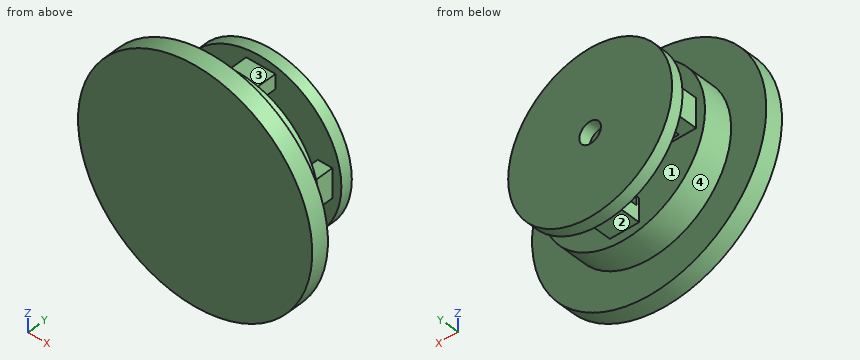
```python
from build123d import *

# Parameters (mm, degrees)
SKETCH_1_R          = 200
EXTRUDE_1_DEPTH     = 30
SKETCH_2_R          = 140
EXTRUDE_2_DEPTH     = 50
SKETCH_4_R          = 1.75
CUT_EXTRUDE_1_DEPTH = 28
SKETCH_7_W          = 25
SKETCH_7_H          = 50
SKETCH_7_W_2        = 50
SKETCH_7_H_2        = 25
EXTRUDE_5_DEPTH     = 43
SKETCH_8_W          = 15
SKETCH_8_H          = 50
SKETCH_8_W_2        = 50
SKETCH_8_H_2        = 15
EXTRUDE_6_DEPTH     = 5
SKETCH_9_R          = 1.75
CUT_EXTRUDE_2_DEPTH = 20
SKETCH_10_R         = 140
EXTRUDE_7_DEPTH     = 20
SKETCH_11_R         = 2.5
CUT_EXTRUDE_3_DEPTH = 20
CUT_EXTRUDE_4_REACH = 318.937
SKETCH_13_R         = 18.5


with BuildPart() as part:
    # 草图1 → 凸台-拉伸1 (new body)
    with BuildSketch(Plane(origin=(0, 0, 0), x_dir=(1, 0, 0), z_dir=(0, 1, 0))):
        with Locations(Location((0, 0, 0), (0, 0, 270))):
            Circle(SKETCH_1_R)
    extrude(amount=EXTRUDE_1_DEPTH)

    # 草图2 → 凸台-拉伸2 (add)
    with BuildSketch(Plane(origin=(0, 30, 0), x_dir=(1, 0, 0), z_dir=(0, 1, 0))):
        with Locations(Location((0, 0, 0), (0, 0, 270))):
            Circle(SKETCH_2_R)
    extrude(amount=EXTRUDE_2_DEPTH)

    # 草图4 → 切除-拉伸1 (cut)
    with BuildSketch(Plane(origin=(0, 80, 0), x_dir=(1, 0, 0), z_dir=(0, 1, 0))):
        with Locations(Location((0, -42.5, 0), (0, 0, 270))):
            Circle(SKETCH_4_R)
        with Locations(Location((-30.0520382, -30.0520382, 0), (0, 0, 270))):
            Circle(SKETCH_4_R)
        with Locations(Location((-42.5, 0, 0), (0, 0, 270))):
            Circle(SKETCH_4_R)
        with Locations(Location((-30.0520382, 30.0520382, 0), (0, 0, 270))):
            Circle(SKETCH_4_R)
        with Locations(Location((0, 42.5, 0), (0, 0, 270))):
            Circle(SKETCH_4_R)
        with Locations(Location((30.0520382, 30.0520382, 0), (0, 0, 270))):
            Circle(SKETCH_4_R)
        with Locations(Location((42.5, 0, 0), (0, 0, 270))):
            Circle(SKETCH_4_R)
        with Locations(Location((30.0520382, -30.0520382, 0), (0, 0, 270))):
            Circle(SKETCH_4_R)
    extrude(amount=-CUT_EXTRUDE_1_DEPTH, mode=Mode.SUBTRACT)

    # 草图7 → 凸台-拉伸5 (add)
    with BuildSketch(Plane(origin=(0, 80, 0), x_dir=(1, 0, 0), z_dir=(0, 1, 0))):
        with Locations((-112.162325809, -2.462481049)):
            Rectangle(SKETCH_7_W, SKETCH_7_H)
        with Locations((2.462481049, -112.162325809)):
            Rectangle(SKETCH_7_W_2, SKETCH_7_H_2)
        with Locations((-2.462481049, 112.162325809)):
            Rectangle(SKETCH_7_W_2, SKETCH_7_H_2)
        with Locations((112.162325809, 2.462481049)):
            Rectangle(SKETCH_7_W, SKETCH_7_H)
    extrude(amount=EXTRUDE_5_DEPTH)

    # 草图8 → 凸台-拉伸6 (add)
    with BuildSketch(Plane(origin=(0, 80, 0), x_dir=(1, 0, 0), z_dir=(0, 1, 0))):
        with Locations((92.162325809, 2.462481049)):
            Rectangle(SKETCH_8_W, SKETCH_8_H)
        with Locations((-2.462481049, 92.162325809)):
            Rectangle(SKETCH_8_W_2, SKETCH_8_H_2)
        with Locations((2.462481049, -92.162325809)):
            Rectangle(SKETCH_8_W_2, SKETCH_8_H_2)
        with Locations((-92.162325809, -2.462481049)):
            Rectangle(SKETCH_8_W, SKETCH_8_H)
    extrude(amount=EXTRUDE_6_DEPTH)

    # 草图9 → 切除-拉伸2 (cut)
    with BuildSketch(Plane(origin=(0, 85, 0), x_dir=(1, 0, 0), z_dir=(0, 1, 0))):
        with Locations(Location((18.656155403, -92.162325809, 0), (0, 0, 270))):
            Circle(SKETCH_9_R)
        with Locations(Location((-11.970984699, -92.162325809, 0), (0, 0, 270))):
            Circle(SKETCH_9_R)
        with Locations(Location((-92.162325809, 11.970984699, 0), (0, 0, 270))):
            Circle(SKETCH_9_R)
        with Locations(Location((-92.162325809, -18.656155403, 0), (0, 0, 270))):
            Circle(SKETCH_9_R)
        with Locations(Location((11.970984699, 92.162325809, 0), (0, 0, 270))):
            Circle(SKETCH_9_R)
        with Locations(Location((-18.656155403, 92.162325809, 0), (0, 0, 270))):
            Circle(SKETCH_9_R)
        with Locations(Location((92.162325809, -11.970984699, 0), (0, 0, 270))):
            Circle(SKETCH_9_R)
        with Locations(Location((92.162325809, 18.656155403, 0), (0, 0, 270))):
            Circle(SKETCH_9_R)
    extrude(amount=-CUT_EXTRUDE_2_DEPTH, mode=Mode.SUBTRACT)

    # 草图10 → 凸台-拉伸7 (add)
    with BuildSketch(Plane(origin=(0, 123, 0), x_dir=(1, 0, 0), z_dir=(0, 1, 0))):
        with Locations(Location((0, 0, 0), (0, 0, 270))):
            Circle(SKETCH_10_R)
    extrude(amount=EXTRUDE_7_DEPTH)

    # 草图11 → 切除-拉伸3 (cut)
    with BuildSketch(Plane(origin=(0, 143, 0), x_dir=(1, 0, 0), z_dir=(0, 1, 0))):
        with Locations(Location((0, 0, 0), (0, 0, 270))):
            Circle(SKETCH_11_R)
    extrude(amount=-CUT_EXTRUDE_3_DEPTH, mode=Mode.SUBTRACT)

    # 草图13 → 切除-拉伸4 (cut, up to next)
    with BuildSketch(Plane(origin=(0, 143, 0), x_dir=(1, 0, 0), z_dir=(0, 1, 0)), mode=Mode.PRIVATE) as cut_extrude_4_sk1:
        with Locations(Location((0, 0, 0), (0, 0, 270))):
            Circle(SKETCH_13_R)
    cut_extrude_4_tool1 = extrude(cut_extrude_4_sk1.sketch, amount=-CUT_EXTRUDE_4_REACH, mode=Mode.PRIVATE) & part.part
    add(cut_extrude_4_tool1.solids().sort_by_distance((0, 143, 0))[0], mode=Mode.SUBTRACT)


solid = part.part
```
Check sheet for the modelled part. Datum: model origin and axes. Units: mm. Face numbers are marked on the shaded views. A direction names the side the tool comes from. Give positions to 0.01 mm unless a question says otherwise; leave off trailing zeros. Loops run counter-clockwise (first coordinate to the right, second up) from the corner with the lowest first, then second, coordinate; pieces in that order, holes last. Notation, with made-up numbers: (18.25, 48.25) - (52.25, 48.25) arc R19 ccw to (52.25, 65.25) - close; hole circle Ø11 at (18, 72.25). An arc over 180 degrees is marked (long way). One line per question, with ' | ' between items. Start each with the question number.
1. Gauge pin test, flat ends, axial feed: pin 1 Ø2.5 at (y, z) = (81.5, 2.5) entering from -X; pin 2 Ø4 at (y, z) = (128.5, 121.5) entering from -X; pin 3 Ø21.5 at (x, y) = (-1, 108.5) entering from +Z. Record the tip position at first contact, or that the pin passes through.
2. Cross-section at A-A, the plane y = 102. Enter the section's corners in (x, z).
3. Cross-section at C-C, the plane x = -54. Enter the section's corners in (y, z).
4. Material ranges on line 1 along Y through (x, z) = (53, -119.5); line 2 along Z through (x, y) = (-23.5, 114.5); line 3 along Y through (x, z) = (-79.5, 155.5), recorded low to high. Write a range as [from, to].
5. Cross-section at B-B, the plane z = -130.5. Enter the section's corners in (x, y), plus the area to 3 significant figures.
6. Cross-section at D-D, the plane y = 45. Enter the section's corners in (x, z), plus the area to 3 significant figures.
7. Set-up check for the marked faces 1, 2, 3 and 4: record each of +Z, -Z, +X, -X, +Y, -Y from which the full face is reachable in a straight line by a thin tool's end or side.
Check result:
1) pin 1: stops at x = -124.66 | pin 2: stops at x = -72.94 | pin 3: stops at z = 124.66
2) outline: (-124.66, -22.54) - (-99.66, -22.54) - (-99.66, 27.46) - (-124.66, 27.46) - close; (-27.46, -124.66) - (22.54, -124.66) - (22.54, -99.66) - (-27.46, -99.66) - close; (-22.54, 99.66) - (27.46, 99.66) - (27.46, 124.66) - (-22.54, 124.66) - close; (99.66, -27.46) - (124.66, -27.46) - (124.66, 22.54) - (99.66, 22.54) - close
3) outline: (0, -192.57) - (30, -192.57) - (30, -129.17) - (80, -129.17) - (80, 129.17) - (30, 129.17) - (30, 192.57) - (0, 192.57) - close; (123, -129.17) - (143, -129.17) - (143, 129.17) - (123, 129.17) - close
4) line 1: y = [0, 80], [123, 143] | line 2: z = [-124.66, -99.66] | line 3: y = [0, 30]
5) outline: (-151.56, 0) - (151.56, 0) - (151.56, 30) - (50.69, 30) - (50.69, 80) - (-50.69, 80) - (-50.69, 30) - (-151.56, 30) - close; (-50.69, 123) - (50.69, 123) - (50.69, 143) - (-50.69, 143) - close | area: 16,200 mm2
6) outline: circle Ø280 at (0, 0) | area: 61,600 mm2
7) face 1: none | face 2: -Z, +X, -X | face 3: +Z, +X, -X | face 4: +Y
